Build history of the part. All positions in model axes, mm. A direction names the side the tool comes from. Coordinates: 2 decimals unless noted, no trailing zeros. Order: outer loops, then holes, each group sorted by start corner. A loop starts at its lowest first (then second) coordinate and runs counter-clockwise, first axis right, second up. Notation, with made-up numbers: (-18.75, -3.75) - (28.25, -3.75) arc R19 cw to (28.25, 12.25) - close; hole circle Ø10 at (79.5, 7.25). An arc over 180 degrees is marked (long way). Write each question's results on one line, items separated by ' | '.
from build123d import *

# Parameters (mm, degrees)
SKETCH_1_W      = 40
SKETCH_1_H      = 9
SKETCH_1_R      = 2
EXTRUDE_1_DEPTH = 4
SKETCH_2_W      = 0.8
SKETCH_2_H      = 9
EXTRUDE_2_DEPTH = 1


with BuildPart() as part:
    # 草图1 → 凸台-拉伸1 (new body)
    with BuildSketch(Plane.XY):
        Rectangle(SKETCH_1_W, SKETCH_1_H)
        Circle(SKETCH_1_R, mode=Mode.SUBTRACT)
    extrude(amount=EXTRUDE_1_DEPTH)

    # 草图2 → 凸台-拉伸2 (add)
    with BuildSketch(Plane.XY.offset(4)):
        with Locations((-19.6, 0)):
            Rectangle(SKETCH_2_W, SKETCH_2_H)
        with Locations((-18, 0)):
            Rectangle(SKETCH_2_W, SKETCH_2_H)
        with Locations((-16.4, 0)):
            Rectangle(SKETCH_2_W, SKETCH_2_H)
        with Locations((16.4, 0)):
            Rectangle(SKETCH_2_W, SKETCH_2_H)
        with Locations((18, 0)):
            Rectangle(SKETCH_2_W, SKETCH_2_H)
        with Locations((19.6, 0)):
            Rectangle(SKETCH_2_W, SKETCH_2_H)
    extrude(amount=EXTRUDE_2_DEPTH)


solid = part.part
1. Probe line 1 (X direction, y = 4.25, z = 4.8); line 2 (Y direction, x = 0, z = 1); line 3 (Z direction, x = -7.5, y = 0.75). List the from-to ranges inside material, lowest first.
Solved:
line 1: x = -20 to -19.2, -18.4 to -17.6, -16.8 to -16, 16 to 16.8, 17.6 to 18.4, 19.2 to 20 | line 2: y = -4.5 to -2, 2 to 4.5 | line 3: z = 0 to 4
2. Drop flat-ended pins along their axis: pin 1 Ø2 at (x, y) = (-13, 0) entering from -Z; pin 2 Ø4.5 at (x, y) = (-2, -2) entering from +Z. Give the stop position or say it passes through.
Solved:
pin 1: stops at z = 0 | pin 2: stops at z = 4
3. Band-saw the part on C-C on y = 0. Give the cut face in (x, z).
Solved:
outline: (-20, 0) - (-2, 0) - (-2, 4) - (-16, 4) - (-16, 5) - (-16.8, 5) - (-16.8, 4) - (-17.6, 4) - (-17.6, 5) - (-18.4, 5) - (-18.4, 4) - (-19.2, 4) - (-19.2, 5) - (-20, 5) - close; (2, 0) - (20, 0) - (20, 5) - (19.2, 5) - (19.2, 4) - (18.4, 4) - (18.4, 5) - (17.6, 5) - (17.6, 4) - (16.8, 4) - (16.8, 5) - (16, 5) - (16, 4) - (2, 4) - close
4. Two-plate mould, pull along Y, no slides. Class faces 1 (the face through (0, 4.5, 2)), 2 (the face through (0, 3, 0)), 3 (the face through (0, -2, 2)): +Y half, -Y half, draft (parallel to the pull), parting line (faces both ways), or undercut.
Solved:
face 1: +Y half | face 2: draft | face 3: undercut
5. Band-saw the part on A-A on z = 4.65. Give the cut face in (x, y), then the cut area to 3 significant figures.
Solved:
outline: (-20, -4.5) - (-19.2, -4.5) - (-19.2, 4.5) - (-20, 4.5) - close; (-18.4, -4.5) - (-17.6, -4.5) - (-17.6, 4.5) - (-18.4, 4.5) - close; (-16.8, -4.5) - (-16, -4.5) - (-16, 4.5) - (-16.8, 4.5) - close; (16, -4.5) - (16.8, -4.5) - (16.8, 4.5) - (16, 4.5) - close; (17.6, -4.5) - (18.4, -4.5) - (18.4, 4.5) - (17.6, 4.5) - close; (19.2, -4.5) - (20, -4.5) - (20, 4.5) - (19.2, 4.5) - close | area: 43.2 mm2
6. Tool access for faces 4 (the face through (-20, 0, 2)), 5 (the face through (17.6, -0.1, 4.5)): list every direction of +Z, -Z, +X, -X, +Y, -Y with a clear straight run to the whole face (end or side of a thin tool).
Solved:
face 4: +Z, -Z, -X, +Y, -Y | face 5: +Z, +Y, -Y
7. Band-saw the part on D-D on x = 14.5. Give the cut face in (y, z), then the cut area to 3 significant figures.
Solved:
outline: (-4.5, 0) - (4.5, 0) - (4.5, 4) - (-4.5, 4) - close | area: 36.0 mm2
8. Band-saw the part on B-B on x = 0. Give the cut face in (y, z).
Solved:
outline: (-4.5, 0) - (-2, 0) - (-2, 4) - (-4.5, 4) - close; (2, 0) - (4.5, 0) - (4.5, 4) - (2, 4) - close
